The listing builds one solid part. Answer for the finished solid, in the listing's coordinates (mm). A direction names the side the tool comes from. Round coordinates to 2 decimals unless told otherwise and drop trailing zeros. Write each loop counter-clockwise with the first axis right and the second up, starting at its lowest first coordinate (ties: lowest second). Pieces come first, ordered by that corner, then holes. Notation, with made-up numbers: (75.25, 88) - (129.25, 88) arc R12 cw to (129.25, 107) - close; hole circle Ø1 at (-8, 31.5). An arc over 180 degrees is marked (long way). Answer in a Markdown table with one row per item.
from build123d import *

# Parameters (mm, degrees)
BOSS_EXTRUDE1_DEPTH             = 103
BOSS_EXTRUDE4_REACH             = 109.274
BOSS_EXTRUDE4_DIRECTION_2_REACH = 109.274
CUT_EXTRUDE1_DEPTH              = 111.752171083
CUT_EXTRUDE1_DEPTH_BACK         = 111.752171083
SKETCH4_R                       = 8
FILLET1_R                       = 3


with BuildPart() as part:
    # Sketch2 → Boss-Extrude1 (new body)
    with BuildSketch(Plane.XY):
        Polygon((-14.529411765, -4.382352941), (-14.529411765, -13.382352941), (18.470588235, -13.382352941), (18.470588235, -4.382352941), (34.470588235, -4.382352941), (34.470588235, 11.617647059), (-30.529411765, 11.617647059), (-30.529411765, -4.382352941), align=None)
    extrude(amount=BOSS_EXTRUDE1_DEPTH)

    # Boss-Extrude4: up to this plane
    boss_extrude4_end = Plane(origin=(34.470588235, 11.617647059, 103), z_dir=(-1, 0, 0))
    # Sketch3 → Boss-Extrude4 (add, up to the surface)
    with BuildSketch(Plane(origin=(-18.747367118, 0, 10.823797452), x_dir=(0, 1, 0), z_dir=(0.866025403784438, 0, -0.500000000000001)), mode=Mode.PRIVATE) as boss_extrude4_sk1:
        with BuildLine():
            Line((11.617647059, 64.814132443), (11.617647059, 26.814132443))
            ThreePointArc((11.617647059, 26.814132443), (30.617647059, 45.814132443), (11.617647059, 64.814132443))
        make_face()
    boss_extrude4_tool1 = split(extrude(boss_extrude4_sk1.sketch, amount=BOSS_EXTRUDE4_REACH, mode=Mode.PRIVATE), bisect_by=boss_extrude4_end, keep=Keep.BOTH, mode=Mode.PRIVATE)
    add(boss_extrude4_tool1.solids().sort_by_distance((4.159699, 19.681498, 50.5))[0])

    # Boss-Extrude4 direction 2: up to this plane
    boss_extrude4_direction_2_end = Plane(origin=(-30.529411765, 11.617647059, 103), z_dir=(1, 0, 0))
    # Sketch3 → Boss-Extrude4 direction 2 (add, up to the surface)
    with BuildSketch(Plane(origin=(-18.747367118, 0, 10.823797452), x_dir=(0, 1, 0), z_dir=(0.866025403784438, 0, -0.500000000000001)), mode=Mode.PRIVATE) as boss_extrude4_direction_2_sk1:
        with BuildLine():
            Line((11.617647059, 64.814132443), (11.617647059, 26.814132443))
            ThreePointArc((11.617647059, 26.814132443), (30.617647059, 45.814132443), (11.617647059, 64.814132443))
        make_face()
    boss_extrude4_direction_2_tool1 = split(extrude(boss_extrude4_direction_2_sk1.sketch, amount=-BOSS_EXTRUDE4_DIRECTION_2_REACH, mode=Mode.PRIVATE), bisect_by=boss_extrude4_direction_2_end, keep=Keep.BOTH, mode=Mode.PRIVATE)
    add(boss_extrude4_direction_2_tool1.solids().sort_by_distance((4.159699, 19.681498, 50.5))[0])

    # Sketch4 → Cut-Extrude1 (cut, two sides: drawn at the far end of the back side and taken through both)
    with BuildSketch(Plane(origin=(-18.747367118, 0, 10.823797452), x_dir=(0, 1, 0), z_dir=(0.866025403784438, 0, -0.500000000000001)).offset(-CUT_EXTRUDE1_DEPTH_BACK)):
        with Locations(Location((11.617647059, 45.814132443, 0), (0, 0, 270))):
            Circle(SKETCH4_R)
    extrude(amount=CUT_EXTRUDE1_DEPTH + CUT_EXTRUDE1_DEPTH_BACK, mode=Mode.SUBTRACT)

    # Fillet1
    fillet1_edges = [part.edges().sort_by_distance(p)[0] for p in [
        (1.970588235, 11.617647059, 73.703193978),
        (1.970588235, 11.617647059, 29.824573519),
    ]]
    fillet(fillet1_edges, radius=FILLET1_R)


solid = part.part
(1) For faces 1 (the flat face through (-23, -4.382, 51)), 2 (the flat face through (10, 11.618, 85)), 3 (the flat face through (-5, 11.618, 17)), 4 (the flat face through (18.471, -9, 51)), determine the directions among +Z, -Z, +X, -X, +Y, -Y from which every point of the face is accessible in a straight line to the end or side of a thin tool.
Checked values:
| item | result |
|---|---|
| face 1 | +Z, -Z, -X, -Y |
| face 2 | +Z, +X, +Y |
| face 3 | -Z, -X, +Y |
| face 4 | +Z, -Z, +X, -Y |
(2) Section A-A (y = 13) is taken. Give the vertices of the cut face in (x, z).
Checked values:
| item | result |
|---|---|
| outline | (-30.53, 48.28) - (34.47, 10.75) - (34.47, 23.9) - (-30.53, 61.43) - close; (-30.53, 79.63) - (34.47, 42.1) - (34.47, 55.25) - (-30.53, 92.78) - close |
(3) For a pull along Z with two mould halves and no side action, classify faces 5 (the flat face through (-30.529, 9, 51)), 6 (the flat face through (2, 2, 103)), 7 (the cylindrical face through (1.9, 19.55, 53.01)) as pulls with the +Z half, pulls with the -Z half, needs draft (parallel to the pull), parting line crosses it, or undercut.
Checked values:
| item | result |
|---|---|
| face 5 | needs draft |
| face 6 | pulls with the +Z half |
| face 7 | undercut |
(4) Find the intervals of material crossed by line 1 (Y direction, x = 29.5, z = 79); line 2 (Z direction, x = -20, y = 17.5); line 3 (Y direction, x = 11, z = 96), in increasing order.
Checked values:
| item | result |
|---|---|
| line 1 | y = -4.38 to 11.62 |
| line 2 | z = 43.59 to 58.19, 70.71 to 85.31 |
| line 3 | y = -13.38 to 11.62 |
(5) Section B-B (y = -9.5) is taken. Give the vertices of the cut face in (x, z).
Checked values:
| item | result |
|---|---|
| outline | (-14.53, 0) - (18.47, 0) - (18.47, 103) - (-14.53, 103) - close |
(6) Section D-D (y = 25) is taken. Give the vertices of the cut face in (x, z), and give its area (3 significant figures).
Checked values:
| item | result |
|---|---|
| outline | (-30.53, 54.95) - (34.47, 17.43) - (34.47, 48.57) - (-30.53, 86.1) - close |
| area | 2,020 mm2 |
(7) Section C-C (y = 18) is taken. Give the vertices of the cut face in (x, z).
Checked values:
| item | result |
|---|---|
| outline | (-30.53, 49.86) - (34.47, 12.34) - (34.47, 27.43) - (-30.53, 64.96) - close; (-30.53, 76.1) - (34.47, 38.57) - (34.47, 53.66) - (-30.53, 91.19) - close |
(8) Flat-ended cylindrical pins translate along their axes: pin 1 (10 mm diameter, centred on x = -5, z = 75, fed in from +Y); pin 2 (2 mm diameter, centred on y = -5.5, z = 82.5, fed in from +X); pin 3 (13 mm diameter, centred on x = 29.5, z = 70.5, fed in from -Y); pin 4 (6 mm diameter, centred on x = 20, y = 10, fed in from -Z). Find the tip coordinate at first contact, or state that the pin passes through.
Checked values:
| item | result |
|---|---|
| pin 1 | stops at y = 26.64 |
| pin 2 | stops at x = 18.47 |
| pin 3 | stops at y = -4.38 |
| pin 4 | stops at z = 0 |
